For this review, use the dimensioned drawing (mm, ordinates from the lowest corner) and the shaded views. A direction names the side the tool comes from. Coordinates: 2 decimals unless noted, no trailing zeros. Write each loop counter-clockwise with the first axis right and the second up, starting at its lowest first coordinate (ties: lowest second). Pieces come first, ordered by that corner, then holes. Notation, with made-up numbers: (-22, -1.5) - (30, -1.5) arc R24 ccw to (30, 34.5) - close; hole circle Ø10 at (-24, 36.25). An arc over 180 degrees is marked (long way). Put each result on its own line as item: value.
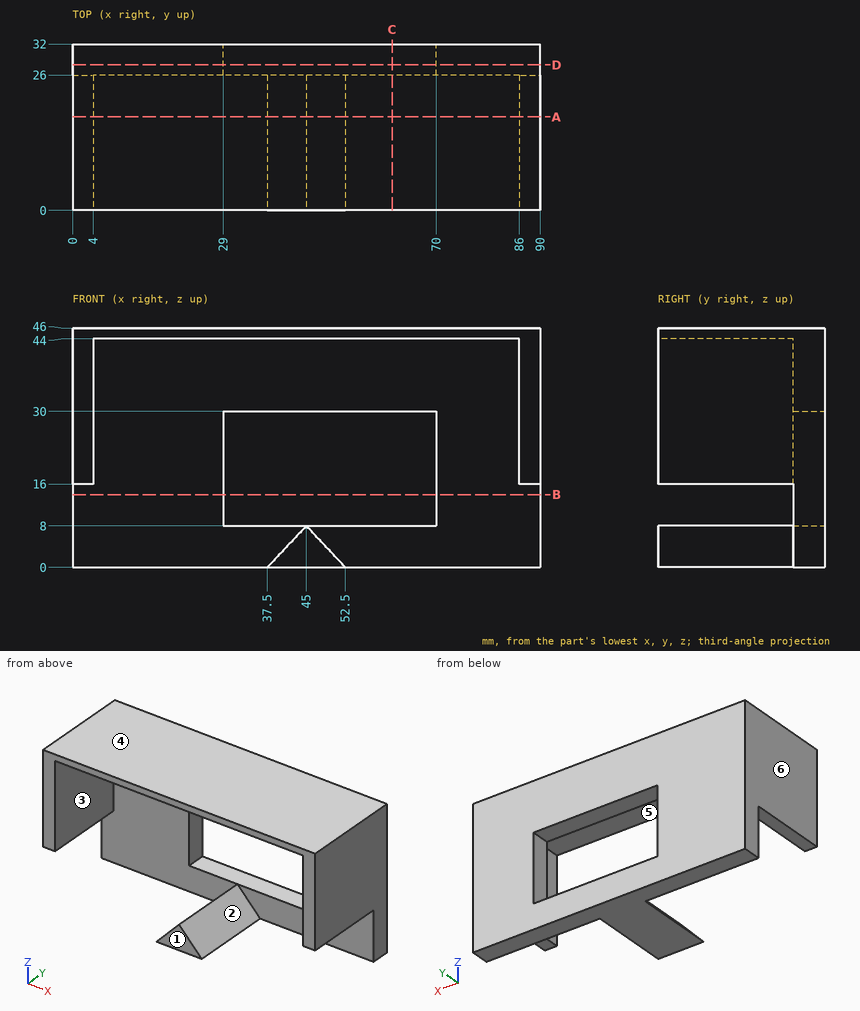
1. To check wall thickness, follow probe 1 along X at (y, z) = (31.5, 18); probe 2 along X at (y, z) = (20, 25); probe 3 along Y at (x, z) = (57, 32.5). State the ranges of each line that lie inside material, in increasing order.
Determined:
probe 1: x = 0 to 29, 70 to 90
probe 2: x = 0 to 4, 86 to 90
probe 3: y = 26 to 32
2. Consider section A-A on y = 18. State the section outline as (x, z) points, plus the area to 3 significant figures.
Determined:
outline: (0, 16) - (4, 16) - (4, 44) - (86, 44) - (86, 16) - (90, 16) - (90, 46) - (0, 46) - close; (37.5, 0) - (52.5, 0) - (45, 8) - close
area: 464 mm^2
3. The part is to be moulded in two halves that separate along X. For the marked faces 4, 5 and 6, say which applies: +X half, -X half, draft (parallel to the pull), parting line (faces both ways), or undercut.
Determined:
face 4: draft
face 5: undercut
face 6: -X half
4. Consider section D-D on y = 28. State the section outline as (x, z) points, plus the area to 3 significant figures.
Determined:
outline: (0, 0) - (90, 0) - (90, 46) - (0, 46) - close; hole (29, 8) - (70, 8) - (70, 30) - (29, 30) - close
area: 3,240 mm^2
5. Machinability: for the marked faces 1, 2 and 3, which of the approach directions +Z, -Z, +X, -X, +Y, -Y give a long, thin tool a straight path to every point of the face, cutting with its end or side? Answer none if there is none.
Determined:
face 1: +Z, -Z, +X, -X, -Y
face 2: +X, -Y
face 3: -Z, -Y
6. Consider section C-C on x = 61.5. State the section outline as (y, z) points, plus the area to 3 significant figures.
Determined:
outline: (0, 44) - (26, 44) - (26, 30) - (32, 30) - (32, 46) - (0, 46) - close; (26, 0) - (32, 0) - (32, 8) - (26, 8) - close
area: 196 mm^2
7. For pin 1 Ø4 at (y, z) = (27.5, 41.5) entering from -X; pin 2 Ø2 at (x, y) = (1.5, 7) entering from -Z; pin 3 Ø5 at (x, z) = (22.5, 28) entering from -Y, all flat-tipped, find the tip position at first contact; note any pin that passes through.
Determined:
pin 1: stops at x = 0
pin 2: stops at z = 16
pin 3: stops at y = 26
8. Consider section B-B on z = 14. State the section outline as (x, y) points, plus the area to 3 significant figures.
Determined:
outline: (0, 26) - (29, 26) - (29, 32) - (0, 32) - close; (70, 26) - (90, 26) - (90, 32) - (70, 32) - close
area: 294 mm^2
